Could you check a few things on this model? Use its own coordinates, in mm. Coordinates: 2 decimals unless noted, no trailing zeros. Loops run counter-clockwise (first coordinate to the right, second up) from the corner with the lowest first, then second, coordinate; pieces in that order, holes last.
from build123d import *

# Parameters (mm, degrees)
BOSS_EXTRUDE1_DEPTH = 3.175
CUT_EXTRUDE1_DEPTH  = 204.138678001
SKETCH3_W           = 42
SKETCH3_H           = 55.35
SKETCH3_W_2         = 30
SKETCH3_H_2         = 80
SKETCH3_W_3         = 7.65
SKETCH3_H_3         = 6.35
CUT_EXTRUDE2_DEPTH  = 204.138678001
FILLET3_R           = 5


with BuildPart() as part:
    # Sketch1 → Boss-Extrude1 (new, symmetric)
    with BuildSketch(Plane(origin=(0, 0, 0), x_dir=(1, 0, 0), z_dir=(0, 1, 0))):
        with BuildLine():
            Line((35, -200), (35, 0))
            ThreePointArc((35, 0), (0, 35), (-35, 0))
            Line((-35, 0), (-35, -200))
            Line((-35, -200), (35, -200))
        make_face()
    extrude(amount=BOSS_EXTRUDE1_DEPTH, both=True)

    # Sketch2 → Cut-Extrude1 (cut, through all)
    with BuildSketch(Plane(origin=(0, 3.175, 0), x_dir=(1, 0, 0), z_dir=(0, 1, 0))):
        with BuildLine():
            Line((-35, -38), (35, -38))
            Line((35, -38), (35, 0))
            ThreePointArc((35, 0), (0, 35), (-35, 0))
            Line((-35, 0), (-35, -38))
        make_face()
    extrude(amount=-CUT_EXTRUDE1_DEPTH, mode=Mode.SUBTRACT)

    # Sketch3 → Cut-Extrude2 (cut, through all)
    with BuildSketch(Plane(origin=(0, 3.175, 0), x_dir=(1, 0, 0), z_dir=(0, 1, 0))):
        with Locations((0, -92.325)):
            Rectangle(SKETCH3_W, SKETCH3_H)
        with Locations((0, -160)):
            Rectangle(SKETCH3_W_2, SKETCH3_H_2)
        with Locations((-24.825, -116.825)):
            Rectangle(SKETCH3_W_3, SKETCH3_H_3)
        with Locations((24.825, -116.825)):
            Rectangle(SKETCH3_W_3, SKETCH3_H_3)
    extrude(amount=-CUT_EXTRUDE2_DEPTH, mode=Mode.SUBTRACT)

    # Fillet3
    fillet3_edges = [part.edges().sort_by_distance(p)[0] for p in [
        (15, 0, 200),
        (-15, 0, 200),
        (35, 0, 200),
        (-35, 0, 200),
    ]]
    fillet(fillet3_edges, radius=FILLET3_R)


solid = part.part
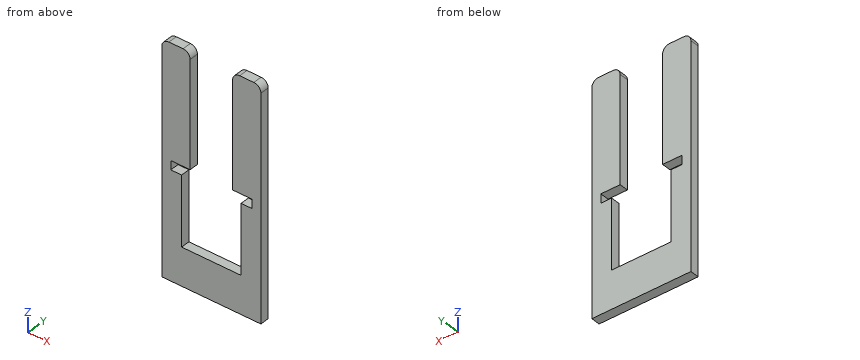
(1) I need wall thicknesses on probe 1 along X at (y, z) = (0, 81); probe 2 along X at (y, z) = (-2.5, 120.5); probe 3 along Z at (x, y) = (28, 2). Which ranges of each line are inside material? Lowest first, please.
Answers:
probe 1: x = -35 to -21, 21 to 35
probe 2: x = -35 to -15, 15 to 35
probe 3: z = 38 to 113.65, 120 to 200
(2) Imagine slicing it at A-A, the plane x = -23.5. Write out the boundary of the cut face in (y, z) (3 decimals).
Answers:
outline: (-3.175, 38) - (3.175, 38) - (3.175, 113.65) - (-3.175, 113.65) - close; (-3.175, 120) - (3.175, 120) - (3.175, 200) - (-3.175, 200) - close
(3) Imagine slicing it at D-D, the plane x = -5. Write out the boundary of the cut face in (y, z) (3 decimals), and give its area (3 significant figures).
Answers:
outline: (-3.175, 38) - (3.175, 38) - (3.175, 64.65) - (-3.175, 64.65) - close
area: 169 mm2
(4) Imagine slicing it at B-B, the plane z = 73. Write out the boundary of the cut face in (x, y) (3 decimals).
Answers:
outline: (-35, -3.175) - (-21, -3.175) - (-21, 3.175) - (-35, 3.175) - close; (21, -3.175) - (35, -3.175) - (35, 3.175) - (21, 3.175) - close
(5) Imagine slicing it at C-C, the plane y = -1.75. Write out the boundary of the cut face in (x, z), and give its area (3 significant figures).
Answers:
outline: (-35, 38) - (35, 38) - (35, 195) arc R5 ccw to (30, 200) - (20, 200) arc R5 ccw to (15, 195) - (15, 120) - (28.65, 120) - (28.65, 113.65) - (21, 113.65) - (21, 64.65) - (-21, 64.65) - (-21, 113.65) - (-28.65, 113.65) - (-28.65, 120) - (-15, 120) - (-15, 195) arc R5 ccw to (-20, 200) - (-30, 200) arc R5 ccw to (-35, 195) - close
area: 6,500 mm2
